from build123d import *

# Parameters (mm, degrees)
EXTRUDE1_DEPTH = 25
SKETCH3_W      = 90
SKETCH3_H      = 50
EXTRUDE2_DEPTH = 10


with BuildPart() as part:
    # Sketch2 → Extrude1 (new body)
    with BuildSketch(Plane.XY):
        Polygon((15, -36.213203436), (15, -56.213203436), (-15, -56.213203436), (-15, -36.213203436), (-36.213203436, -15), (-36.213203436, 15), (-15, 36.213203436), (15, 36.213203436), (36.213203436, 15), (36.213203436, -15), align=None)
    extrude(amount=EXTRUDE1_DEPTH)

    # Sketch3 → Extrude2 (add)
    with BuildSketch(Plane.XZ.offset(56.213203436)):
        Rectangle(SKETCH3_W, SKETCH3_H)
    extrude(amount=EXTRUDE2_DEPTH)


solid = part.part
Work out the finished part from the listing and answer in its coordinate system (mm). A direction names the side the tool comes from. Give positions to 0.01 mm unless a question says otherwise; leave off trailing zeros. Write each loop counter-clockwise with the first axis right and the second up, starting at its lowest first coordinate (ties: lowest second). Pieces come first, ordered by that corner, then holes. Notation, with made-up numbers: (75.25, -22) - (132.25, -22) arc R21 cw to (132.25, -2) - close; hole circle Ø9 at (-27.75, 64). An arc over 180 degrees is marked (long way). One line per item, written item: value. Start each with the question number.
1. For faces 4 (the flat face through (1, 1, 0)), 5 (the flat face through (15, -46, 12)), 6 (the flat face through (-36.213, 0, 12)), 7 (the flat face through (-1, -56.213, -5)), determine the directions among +Z, -Z, +X, -X, +Y, -Y from which every point of the face is accessible in a straight line to the end or side of a thin tool.
2. Find section A-A (x = 32). Write down the section's boundary in (y, z).
3. Consider probe 1 along Y at (x, z) = (-15, -1.5); probe 2 along Z at (x, y) = (20, 28); probe 3 along X at (y, z) = (9.5, 17.5). Determine where each line is inside the solid, lowest interval first.
4. Find section B-B (z = 7). Write down the section's boundary in (x, y).
5. Find section D-D (x = -4). Write down the section's boundary in (y, z).
6. For a pull along Y with two mould halves and no side action, classify faces 1 (the flat face through (-45, -61, 0)), 2 (the flat face through (-25.458, -25.755, 12.325)), 3 (the flat face through (-1, -66.213, 0)) as +Y half, -Y half, draft (parallel to the pull), parting line (faces both ways), or undercut.
7. Given pin 1 (3 mm diameter, centred on x = 28, z = -12.5, fed in from +Y); pin 2 (1.5 mm diameter, centred on x = -8, y = -28, fed in from -Z); pin 3 (22 mm diameter, centred on y = -44.5, z = 16, fed in from +X), each flat-ended and moving along its own axis, determine where each tip first touches the part or whether it passes through.
8. Find section C-C (y = -44). Write down the section's boundary in (x, z), then the cut area to 3 significant figures.
Geometry results:
1. face 4: -Z, +X, -X, +Y
1. face 5: +Z, -Z, +X
1. face 6: +Z, -Z, -X, +Y
1. face 7: -Z
2. outline: (-66.21, -25) - (-56.21, -25) - (-56.21, 25) - (-66.21, 25) - close; (-19.21, 0) - (19.21, 0) - (19.21, 25) - (-19.21, 25) - close
3. probe 1: -66.21 to -56.21
3. probe 2: 0 to 25
3. probe 3: -36.21 to 36.21
4. outline: (-45, -66.21) - (45, -66.21) - (45, -56.21) - (15, -56.21) - (15, -36.21) - (36.21, -15) - (36.21, 15) - (15, 36.21) - (-15, 36.21) - (-36.21, 15) - (-36.21, -15) - (-15, -36.21) - (-15, -56.21) - (-45, -56.21) - close
5. outline: (-66.21, -25) - (-56.21, -25) - (-56.21, 0) - (36.21, 0) - (36.21, 25) - (-66.21, 25) - close
6. face 1: draft
6. face 2: undercut
6. face 3: -Y half
7. pin 1: y = -56.21
7. pin 2: z = 0
7. pin 3: x = 17.71
8. outline: (-15, 0) - (15, 0) - (15, 25) - (-15, 25) - close
8. area: 750 mm2
